Part model, mm, in its own coordinate system. Face numbers are marked on the shaded views. A direction names the side the tool comes from. Round coordinates to 2 decimals unless told otherwise and drop trailing zeros. Loops run counter-clockwise (first coordinate to the right, second up) from the corner with the lowest first, then second, coordinate; pieces in that order, holes last. Notation, with made-up numbers: (13, 28) -> (30, 28) arc R28 cw to (30, 63) -> close; hole circle Ø11 at (86, -1). An arc over 180 degrees is marked (long way). Use a Markdown table: item, result. Add a question column.
Item 1: Cut at B-B, the plane z = 14.5. List the corners of the cut face in (x, y), plus the area to 3 significant figures.
Item 2: Which spindle directions (+Z, -Z, +X, -X, +Y, -Y) get a long thin tool onto all of the face, cutting with end or side? Do the marked faces 1 and 2. Say none if no direction does.
Item 3: Cut at D-D, the plane y = -24. List the corners of the cut face in (x, z), plus the area to 3 significant figures.
Item 4: Flat gauge pins, fed straight in: pin 1 (12 mm diameter, centred on x = -6.5, z = 16.5, fed in from -Y); pin 2 (6 mm diameter, centred on x = -4.5, z = 22.5, fed in from -Y); pin 3 (1 mm diameter, centred on x = -20.5, y = -21.5, fed in from -Z). Where does each tip first touch, or does it go through?
Item 5: Probe line 1 (Z direction, x = -6.5, y = -22.5); line 2 (Y direction, x = -2.5, z = 8); line 3 (Y direction, x = -2.25, z = 21.5). List the from-to ranges inside material, lowest first. Write a range as [from, to].
Item 6: Two-plate mould, pull along Z, no slides. Class the marked faces 3, 4 and 5: pulls with the +Z half, pulls with the -Z half, needs draft (parallel to the pull), parting line crosses it, or undercut.
Item 7: Cut at A-A, the plane y = -16. List the corners of the cut face in (x, z).
Item 8: Cut at C-C, the plane x = -12.25. List the corners of the cut face in (y, z).
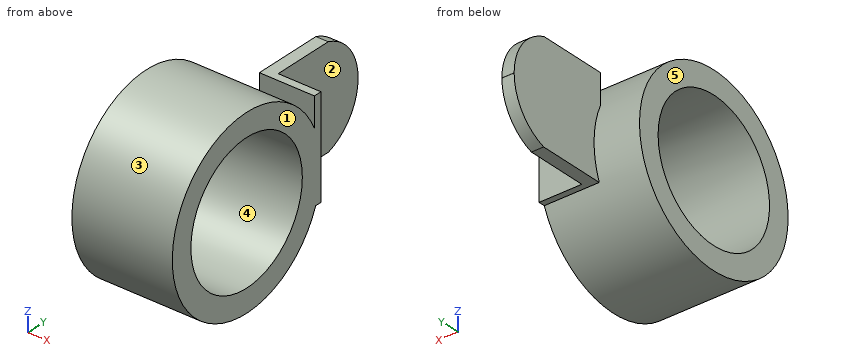
```python
from build123d import *

# Parameters (mm, degrees)
F1_DEPTH = 25
F3_DEPTH = 25
F4_R     = 22.7224143994
F4_R_2   = 17.0375954798
F5_DEPTH = 25


# Not quite as in the source:
# - ends of sketch curves that miss each other by under 0.0002 mm in the source are joined


with BuildPart() as f1:
    # F0 (on Top) → F1 (new body)
    with BuildSketch(Plane.XY):
        Polygon((0, 0), (-10.6365969405, 0), (-10.6365969405, 24.4365315884), (-13.6861931533, 24.4365315884), (-13.6861931533, 0), (-13.6861931533, -2), (0, -2), align=None)
    extrude(amount=F1_DEPTH)

    # F2 (on face) → F3 (cut)
    with BuildSketch(Plane.YZ.offset(-10.6365969405)):
        with BuildLine():
            ThreePointArc((24.4365498995, 12.4780622919), (21.9456846424, 4.7798806359), (15.4173501195, 0))
            Line((15.4173501195, 0), (24.4365315884, 0))
            Line((24.4365315884, 0), (24.4365498995, 12.4780622919))
        make_face()
        with BuildLine():
            ThreePointArc((15.2820812933, 25), (21.9038763933, 20.233757287), (24.4365498995, 12.4780622919))
            Line((24.4365498995, 12.4780622919), (24.4365315884, 25))
            Line((24.4365315884, 25), (15.2820812933, 25))
        make_face()
    extrude(amount=-F3_DEPTH, mode=Mode.SUBTRACT)

    # F4 (on Right) → F5 (join)
    with BuildSketch(Plane.YZ):
        with Locations((-22.7224143994, 8.3613144234)):
            Circle(F4_R)
        with Locations((-22.7224143994, 8.3613144234)):
            Circle(F4_R_2, mode=Mode.SUBTRACT)
    extrude(amount=-F5_DEPTH)


solid = f1.part
```
A:
| question | item | result |
|---|---|---|
| 1 | outline | (-25, -44.6) -> (0, -44.6) -> (0, -38.62) -> (-25, -38.62) -> close; (-25, -6.83) -> (0, -6.83) -> (0, 0) -> (-10.64, 0) -> (-10.64, 24.28) -> (-13.69, 24.28) -> (-13.69, -0.84) -> (-25, -0.84) -> close |
| 1 | area | 385 mm^2 |
| 2 | face 1 | +Z, -Z, +X, +Y, -Y |
| 2 | face 2 | +Z, -Z, +X, +Y |
| 3 | outline | (-25, -14.33) -> (0, -14.33) -> (0, -8.63) -> (-25, -8.63) -> close; (-25, 25.35) -> (0, 25.35) -> (0, 31.05) -> (-25, 31.05) -> close |
| 3 | area | 285 mm^2 |
| 4 | pin 1 | stops at y = -45.34 |
| 4 | pin 2 | stops at y = -42.53 |
| 4 | pin 3 | stops at z = -14.35 |
| 5 | line 1 | z = [-14.36, -8.67], [25.4, 31.08] |
| 5 | line 2 | y = [-45.44, -39.76], [-5.69, 0] |
| 5 | line 3 | y = [-41.26, -33.57], [-11.88, -4.18], [-2, 0] |
| 6 | face 3 | parting line crosses it |
| 6 | face 4 | undercut |
| 6 | face 5 | needs draft |
| 7 | outline | (-25, -13.34) -> (0, -13.34) -> (0, -7.29) -> (-25, -7.29) -> close; (-25, 24.02) -> (0, 24.02) -> (0, 30.07) -> (-25, 30.07) -> close |
| 8 | outline | (-2, 17.68) arc R22.72 ccw (long way) to (-1.59, 0) -> (15.42, 0) arc R13.14 ccw to (24.44, 12.46) -> (24.44, 12.5) arc R13.14 ccw to (15.28, 25) -> (-2, 25) -> close; hole circle Ø34.08 at (-22.72, 8.36) |
